Here's how the part is built. I have some questions about the finished solid (model axes, mm). Face numbers are marked on the shaded views. Coordinates: 2 decimals unless noted, no trailing zeros. Order: outer loops, then holes, each group sorted by start corner. A loop starts at its lowest first (then second) coordinate and runs counter-clockwise, first axis right, second up. Notation, with made-up numbers: (80.5, 26.5) - (94.5, 26.5) arc R19 ccw to (94.5, 59.5) - close; hole circle Ø4 at (55.25, -28.5). An arc over 180 degrees is marked (long way). Use one line per item in the form item = value. Start each with the question number.
Autodesk Inventor part; units mm, degrees
ref_plane "YZ Plane" through (0, 0, 0) normal (1, 0, 0) x (0, 1, 0)
ref_plane "XZ Plane" through (0, 0, 0) normal (0, 1, 0) x (-1, 0, 0)
ref_plane "XY Plane" through (0, 0, 0) normal (0, 0, 1) x (1, 0, 0)
sketch "Sketch1" plane through (0, 0, 0) normal (0, 0, 1) x (1, 0, 0)
  line L0 (-51.9238, 7.67) -> (40.5487, 7.67)
  line L1 (50.9762, -5.53) -> (50.9762, -7.53)
  line L2 (50.9762, -7.53) -> (-51.9238, -7.53)
  line L3 (-51.9238, -7.53) -> (-51.9238, 7.67)
  line L4 (-51.9238, 7.67) -> (50.9762, -7.53) construction
  line L5 (50.8142, 7.3691) -> (-51.9238, -7.53) construction
  line L6 (40.55, -5.53) -> (50.9762, -5.53)
  line L7 (40.5487, 5.67) -> (-49.9238, 5.67)
  line L8 (-49.9238, 5.67) -> (-49.9238, 3.42)
  line L9 (-49.9238, 3.42) -> (38.3707, 3.42)
  line L10 (40.5487, 7.67) -> (40.5487, 5.8804)
  line L11 (40.55, -5.53) -> (-49.9238, -5.53)
  line L12 (-49.9238, -5.53) -> (-49.9238, -3.28)
  line L13 (-49.9238, -3.28) -> (38.3707, -3.28)
  line L14 (40.5487, 5.8804) -> (40.5487, 5.67)
  line L15 (38.3707, 2.82) -> (-49.9238, 2.82)
  line L16 (-49.9238, 2.82) -> (-49.9238, 0.57)
  line L17 (-49.9238, 0.57) -> (38.3707, 0.57)
  line L18 (38.3707, 3.42) -> (38.3707, 2.82)
  line L19 (38.3707, -0.03) -> (-49.9238, -0.03)
  line L20 (-49.9238, -0.03) -> (-49.9238, -2.28)
  line L21 (-49.9238, -2.28) -> (38.3707, -2.28)
  line L22 (38.3707, 0.57) -> (38.3707, -0.03)
  line L23 (38.3707, -2.28) -> (38.3707, -3.28)
  point P0 (0, 0)
  dimension "d0" = 102.9
  dimension "d1" = 14.9
  dimension "d3" = 2
  dimension "d4" = 2
  dimension "d5" = 2.25
  dimension "d6" = 2
  dimension "d7" = 2
  dimension "d8" = 2.25
  dimension "d10" = 0.6
  dimension "d11" = 2.25
  dimension "d12" = 2
  dimension "d13" = 0.6
  dimension "d14" = 2.25
  dimension "d15" = 1
  dimension "d16" = 2
extrude "Extrusion1" add sketch "Sketch1" along normal blind 54.5
sketch "Sketch2" plane through (0, 0, 54.5) normal (0, 0, 1) x (1, 0, 0)
  line L0 (-51.9238, 7.67) -> (40.5487, 7.67)
  line L1 (50.9762, -7.53) -> (-51.9238, -7.53)
  line L2 (40.5487, 7.67) -> (-51.9238, 7.67)
  line L3 (-51.9238, 7.67) -> (-51.9238, -7.53)
  line L4 (-51.9238, -7.53) -> (40.5487, -7.53)
  line L5 (40.5487, -7.53) -> (40.5487, 7.67)
  point P0 (0, 0)
extrude "Extrusion2" add sketch "Sketch2" along normal blind 2
sketch "Sketch3" plane through (0, 0, 0) normal (0, 0, -1) x (-1, 0, 0)
  line L0 (-40.5487, 7.67) -> (-40.5487, 5.67)
  line L1 (51.9238, -7.53) -> (51.9238, 7.67)
  line L2 (-40.5487, 7.67) -> (51.9238, 7.67)
  line L3 (51.9238, 7.67) -> (51.9238, -7.53)
  line L4 (51.9238, -7.53) -> (-40.5487, -7.53)
  line L5 (-40.5487, -7.53) -> (-40.5487, 7.67)
  point P0 (0, 0)
extrude "Extrusion3" add sketch "Sketch3" along normal blind 2
sketch "Sketch4" plane through (40.5487, -7.53, 0) normal (0, -1, 0) x (1, 0, 0)
  line L0 (8.4275, 31.25) -> (2.4275, 31.25)
  line L1 (2.4275, 31.25) -> (2.4275, 23.25)
  line L2 (2.4275, 23.25) -> (8.4275, 23.25)
  line L3 (8.4275, 23.25) -> (8.4275, 31.25)
  line L4 (10.4275, 0) -> (10.4275, 54.5)
  line L5 (10.4275, 0) -> (0, 0)
  point P0 (-40.5487, 0)
  dimension "d23" = 2
  dimension "d24" = 8
  dimension "d25" = 6
  dimension "d26" = 23.25
extrude "Extrusion4" cut sketch "Sketch4" against normal blind 2
properties part number "CardBox_4slots"
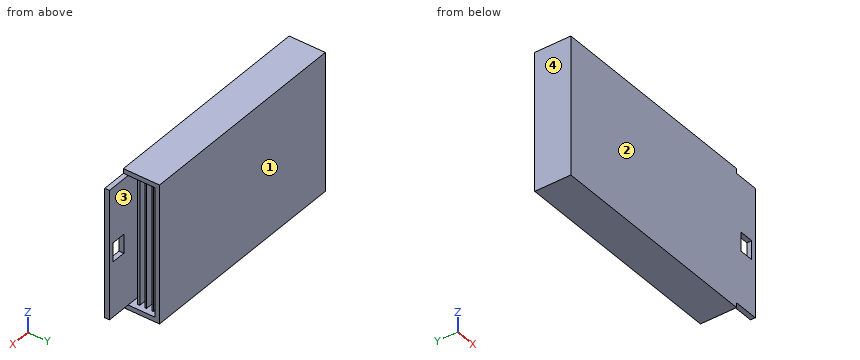
1) Suppose I cut it at B-B, the plane x = -7. List the corners of the cut face in (y, z) for me, then the cut area to 3 significant figures.
2) For pin 1 (6 mm diameter, centred on y = 5.5, z = 49.5, fed in from +X); pin 2 (0.7 mm diameter, centred on y = -5, z = 30, fed in from +X); pin 3 (1.6 mm diameter, centred on x = 47, y = -6.5, fed in from -Z), each with a flat end and sliding along its axis, tell me the tip position at first contact or that it passes through.
3) Suppose I cut it at C-C, the plane y = -1. List the corners of the cut face in (x, z) for me.
4) Suppose I cut it at D-D, the plane z = 19. List the corners of the cut face in (x, y) for me.
5) I need wall thicknesses on probe 1 along Y at (x, z) = (1, 8); probe 2 along Z at (x, y) = (-4.5, -5.5); probe 3 along X at (y, z) = (-6.5, 25.5). Which ranges of each line are inside material? Lowest first, please. Write a range as [from, to].
6) Suppose I cut it at A-A, the plane z = 28. List the corners of the cut face in (x, y) for me, then the cut area to 3 significant figures.
7) If we mould it in two halves opening along Y, with no side actions, what happens to the marked faces 1, 2, 3 and 4? For each: pulls with the +Y half, pulls with the -Y half, needs draft (parallel to the pull), parting line crosses it, or undercut.
From the geometry:
q1.outline = (-7.53, -2) - (7.67, -2) - (7.67, 56.5) - (-7.53, 56.5) - close; hole (-5.53, 0) - (-3.28, 0) - (-3.28, 54.5) - (-5.53, 54.5) - close; hole (-2.28, 0) - (-0.03, 0) - (-0.03, 54.5) - (-2.28, 54.5) - close; hole (0.57, 0) - (2.82, 0) - (2.82, 54.5) - (0.57, 54.5) - close; hole (3.42, 0) - (5.67, 0) - (5.67, 54.5) - (3.42, 54.5) - close
q1.area = 399 mm2
q2.pin_1 = 40.55
q2.pin_2 = -49.92
q2.pin_3 = 0
q3.outline = (-51.92, -2) - (40.55, -2) - (40.55, 0) - (-49.92, 0) - (-49.92, 54.5) - (40.55, 54.5) - (40.55, 56.5) - (-51.92, 56.5) - close
q4.outline = (-51.92, -7.53) - (50.98, -7.53) - (50.98, -5.53) - (-49.92, -5.53) - (-49.92, -3.28) - (38.37, -3.28) - (38.37, -2.28) - (-49.92, -2.28) - (-49.92, -0.03) - (38.37, -0.03) - (38.37, 0.57) - (-49.92, 0.57) - (-49.92, 2.82) - (38.37, 2.82) - (38.37, 3.42) - (-49.92, 3.42) - (-49.92, 5.67) - (40.55, 5.67) - (40.55, 7.67) - (-51.92, 7.67) - close
q5.probe_1 = [-7.53, -5.53], [-3.28, -2.28], [-0.03, 0.57], [2.82, 3.42], [5.67, 7.67]
q5.probe_2 = [-2, 0], [54.5, 56.5]
q5.probe_3 = [-51.92, 42.98], [48.98, 50.98]
q6.outline = (-51.92, -7.53) - (42.98, -7.53) - (42.98, -5.53) - (-49.92, -5.53) - (-49.92, -3.28) - (38.37, -3.28) - (38.37, -2.28) - (-49.92, -2.28) - (-49.92, -0.03) - (38.37, -0.03) - (38.37, 0.57) - (-49.92, 0.57) - (-49.92, 2.82) - (38.37, 2.82) - (38.37, 3.42) - (-49.92, 3.42) - (-49.92, 5.67) - (40.55, 5.67) - (40.55, 7.67) - (-51.92, 7.67) - close; (48.98, -7.53) - (50.98, -7.53) - (50.98, -5.53) - (48.98, -5.53) - close
q6.area = 595 mm2
q7.face_1 = pulls with the +Y half
q7.face_2 = pulls with the -Y half
q7.face_3 = undercut
q7.face_4 = needs draft
